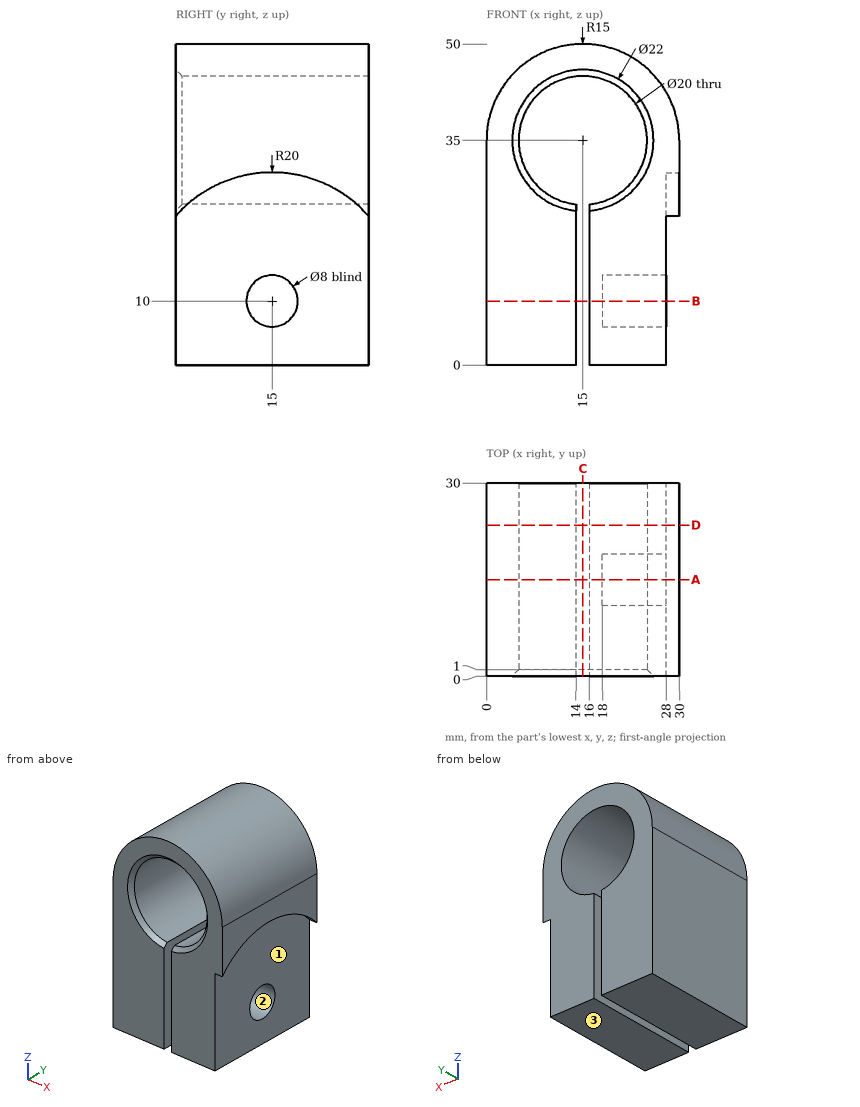
Answer from the drawing. Dimensions are ordinates in mm from the lowest x, y and z of the part. Round coordinates to 2 decimals unless told otherwise and drop trailing zeros. Write each loop counter-clockwise with the first axis right and the second up, starting at its lowest first coordinate (ties: lowest second). Pieces come first, ordered by that corner, then holes. Notation, with made-up numbers: (82, 41.25) -> (130, 41.25) arc R19 cw to (130, 45.25) -> close; hole circle Ø3 at (-26, 62). An arc over 180 degrees is marked (long way). Answer in a Markdown table with one row per item. Add a question column.
1) Find section B-B, the plane z = 10. Determine the outline of the cut face in (x, y).
2) Consider line 1 (X direction, y = 28.75, z = 14); line 2 (Z direction, x = 23, y = 15); line 3 (Z direction, x = 19.25, y = 12). Determine where each line is inside the solid, lowest interval first.
3) Determine the mould class of the marked faces 1, 2 and 3 for opening direction Z: pulls with the +Z half, pulls with the -Z half, needs draft (parallel to the pull), parting line crosses it, or undercut.
4) Find section A-A, the plane y = 15. Determine the outline of the cut face in (x, z), and give its area (3 significant figures).
5) Find section C-C, the plane x = 15. Determine the outline of the cut face in (y, z).
6) Given P1, Ø15, axis at y = 20, z = 19, coming from the +X side; P2, Ø2.5, axis at y = 15.5, z = 10.5, coming from the +X side; P3, Ø1.5, axis at y = 4, z = 41, coming from the +X side; P4, Ø16, axis at x = 15, z = 35, coming from the -Y side, each flat-ended and moving along its own axis, determine where each tip first touches the part or whether it passes through.
7) Find section D-D, the plane y = 23.5. Determine the outline of the cut face in (x, z).
Findings below:
| question | item | result |
|---|---|---|
| 1 | outline | (0, 0) -> (14, 0) -> (14, 30) -> (0, 30) -> close; (16, 0) -> (28, 0) -> (28, 11) -> (18, 11) -> (18, 19) -> (28, 19) -> (28, 30) -> (16, 30) -> close |
| 2 | line 1 | 0 to 14, 16 to 28 |
| 2 | line 2 | 0 to 6, 14 to 29, 41 to 47.69 |
| 2 | line 3 | 0 to 7.35, 12.65 to 25.95, 44.05 to 49.39 |
| 3 | face 1 | needs draft |
| 3 | face 2 | undercut |
| 3 | face 3 | pulls with the -Z half |
| 4 | outline | (0, 0) -> (14, 0) -> (14, 25.05) arc R10 cw (long way) to (16, 25.05) -> (16, 0) -> (28, 0) -> (28, 6) -> (18, 6) -> (18, 14) -> (28, 14) -> (28, 30) -> (30, 30) -> (30, 35) arc R15 ccw to (0, 35) -> close |
| 4 | area | 899 mm² |
| 5 | outline | (0, 46) -> (1, 45) -> (30, 45) -> (30, 50) -> (0, 50) -> close |
| 6 | P1 | x = 28 |
| 6 | P2 | x = 18 |
| 6 | P3 | x = 29.05 |
| 6 | P4 | through |
| 7 | outline | (0, 0) -> (14, 0) -> (14, 25.05) arc R10 cw (long way) to (16, 25.05) -> (16, 0) -> (28, 0) -> (28, 28.1) -> (30, 28.1) -> (30, 35) arc R15 ccw to (0, 35) -> close |
